Could you check a few things on this model? Use its own coordinates, in mm. A direction names the side the tool comes from. Give positions to 0.01 mm unless a question says otherwise; leave off trailing zeros. Loops run counter-clockwise (first coordinate to the right, second up) from the corner with the lowest first, then second, coordinate; pieces in that order, holes last. Notation, with made-up numbers: (87.5, 31.5) -> (134.5, 31.5) arc R29 cw to (134.5, 58.5) -> close; hole circle Ø8 at (34, -11.5). An arc over 180 degrees is marked (long way). Write each question's results on one line, items separated by ' | '. Start each with the question number.
Q1. Which directions (+Z, -Z, +X, -X, +Y, -Y) give clear straight access to the entire face, cutting with the end or side of a thin tool? Please do faces 4 (the face through (-1, -15, 52.754)), 5 (the face through (-28.086, -9, 0)), 6 (the face through (0, -72.807, 41)).
Q2. If I drill on line 1 along X through (y, z) = (-20, -14); line 2 along Y through (x, z) = (31, 22); line 3 along X through (y, z) = (-7, -22), over which ranges is the centre line in solid material (lowest first)?
Q3. If we section it at D-D, the plane y = -15: List the corners of the cut face in (x, z) for me, plus the area to 3 significant figures.
Q4. If we section it at B-B, the plane y = -47.5: List the corners of the cut face in (x, z) for me.
Q5. We'd pull the mould along X, two halves only. Please class faces 1 (the face through (28.086, -9, 0)), 2 (the face through (56.194, -25, 23)), 3 (the face through (-56.194, -25, 23)): released by +X, released by -X, zero draft, split by the parting line, or undercut.
Q6. Will these pins go through, and if not, where does the flat tip stop? P1, Ø3, axis at x = -37.5, y = -32.5, coming from the -Z side; P2, Ø6, axis at x = -39.5, y = -19.5, coming from the -Z side; P3, Ø9, axis at x = -11.5, y = -5, coming from the -Z side.
Q7. If we section it at C-C, the plane z = 14: List the corners of the cut face in (x, y) for me.
Q8. If we section it at A-A, the plane x = -1: List the corners of the cut face in (y, z) for me.
from build123d import *

# Parameters (mm, degrees)
F0_W     = 112.387598
F0_H     = 105.508096
F0_W_2   = 56.171656
F0_H_2   = 52.476138
F1_DEPTH = 93.251504
F3_DEPTH = 50000
F4_W     = 62.165468
F4_H     = 54.584294
F5_DEPTH = 105.509097


with BuildPart() as f1:
    # F0 (on Front) → F1 (new body)
    with BuildSketch(Plane.XZ):
        Rectangle(F0_W, F0_H)
        Rectangle(F0_W_2, F0_H_2, mode=Mode.SUBTRACT)
    extrude(amount=F1_DEPTH)

    # F2 (on face) → F3 (cut, symmetric)
    with BuildSketch(Plane(origin=(-56.193799, 0, 0), x_dir=(0, -1, 0), z_dir=(-1, 0, 0))):
        Polygon((93.251504, 52.754048), (0, -52.754048), (93.251504, -52.754048), align=None)
    extrude(amount=F3_DEPTH, both=True, mode=Mode.SUBTRACT)

    # F4 (on face) → F5 (cut, through all)
    with BuildSketch(Plane.XY.offset(52.754048)):
        with Locations((0, -45.515299)):
            Rectangle(F4_W, F4_H)
    extrude(amount=-F5_DEPTH, mode=Mode.SUBTRACT)


solid = f1.part
Final values:
1) face 4: +Z, +X, -X, +Y, -Y | face 5: +Y, -Y | face 6: +Z, -Z
2) line 1: x = -56.19 to -31.08, 31.08 to 56.19 | line 2: y = -18.22 to 0 | line 3: x = -56.19 to -28.09, 28.09 to 56.19
3) outline: (-56.19, -35.78) -> (56.19, -35.78) -> (56.19, 52.75) -> (-56.19, 52.75) -> close; hole (-28.09, -26.24) -> (28.09, -26.24) -> (28.09, 26.24) -> (-28.09, 26.24) -> close | area: 7,000 mm²
4) outline: (-56.19, 0.99) -> (-31.08, 0.99) -> (-31.08, 52.75) -> (-56.19, 52.75) -> close; (31.08, 0.99) -> (56.19, 0.99) -> (56.19, 52.75) -> (31.08, 52.75) -> close
5) face 1: undercut | face 2: released by +X | face 3: released by -X
6) P1: stops at z = -17.68 | P2: stops at z = -34.09 | P3: stops at z = -52.19
7) outline: (-56.19, -59) -> (-31.08, -59) -> (-31.08, -18.22) -> (-28.09, -18.22) -> (-28.09, 0) -> (-56.19, 0) -> close; (28.09, -18.22) -> (31.08, -18.22) -> (31.08, -59) -> (56.19, -59) -> (56.19, 0) -> (28.09, 0) -> close
8) outline: (-93.25, 52.75) -> (-72.81, 29.62) -> (-72.81, 52.75) -> close; (-18.22, -32.14) -> (0, -52.75) -> (0, -26.24) -> (-18.22, -26.24) -> close; (-18.22, 26.24) -> (0, 26.24) -> (0, 52.75) -> (-18.22, 52.75) -> close
